from build123d import *

# Parameters (mm, degrees)
SKETCH1_W           = 186.97
SKETCH1_H           = 23
BOSS_EXTRUDE1_DEPTH = 4
SKETCH2_W           = 10
SKETCH2_H           = 23
BOSS_EXTRUDE2_DEPTH = 22
BOSS_EXTRUDE3_DEPTH = 8
CHAMFER1_SIZE       = 14.301043111
CHAMFER1_SIZE_2     = 12
CUT_EXTRUDE1_REACH  = 191.66
SKETCH4_W           = 9
SKETCH4_H           = 4.8
SKETCH4_H_2         = 4
SKETCH4_H_3         = 2.2
SKETCH4_W_2         = 3
SKETCH4_H_4         = 3
SKETCH5_W           = 6
SKETCH5_H           = 6
BOSS_EXTRUDE4_DEPTH = 9
CUT_EXTRUDE2_REACH  = 191.66
SKETCH6_W           = 6
SKETCH6_H           = 4
CUT_EXTRUDE3_REACH  = 192.165
SKETCH7_W           = 3
SKETCH7_H           = 3
SKETCH8_W           = 16
SKETCH8_H           = 23
BOSS_EXTRUDE5_DEPTH = 14
CHAMFER2_SIZE       = 14
CHAMFER2_SIZE_2     = 16.105157701
SKETCH9_W           = 9
SKETCH9_H           = 9
CUT_EXTRUDE4_DEPTH  = 2


with BuildPart() as part:
    # Sketch1 → Boss-Extrude1 (new body)
    with BuildSketch(Plane(origin=(0, 0, 0), x_dir=(1, 0, 0), z_dir=(0, 1, 0))):
        with Locations((93.485, 11.5)):
            Rectangle(SKETCH1_W, SKETCH1_H)
    extrude(amount=BOSS_EXTRUDE1_DEPTH)

    # Sketch2 → Boss-Extrude2 (add)
    with BuildSketch(Plane.XZ):
        with Locations((172.97, -11.5)):
            Rectangle(SKETCH2_W, SKETCH2_H)
    extrude(amount=BOSS_EXTRUDE2_DEPTH)

    # Sketch3 → Boss-Extrude3 (add)
    with BuildSketch(Plane.XZ):
        Polygon((167.97, 0), (38.01, 0), (38.01, -8), (38.01, -23), (62.01, -23), (62.01, -8), (167.97, -8), align=None)
    extrude(amount=BOSS_EXTRUDE3_DEPTH)

    # Chamfer1
    # the kernel refuses this chamfer: 14.301043111, 12 mm, written as the material it adds along each edge
    with BuildSketch(Plane(origin=(167.97, -8, -8), x_dir=(0.024939322090235156, -0.9996889667359941, 0), z_dir=(0, 0, 1))) as chamfer1_piece_1_section:
        Polygon((CHAMFER1_SIZE * 0.999688966745, -CHAMFER1_SIZE * 0.0249393220905), (-CHAMFER1_SIZE_2 * 0.0249393220902, -CHAMFER1_SIZE_2 * 0.999688966736), (0, 0), align=None)
    chamfer1_piece_1 = extrude(amount=8, mode=Mode.PRIVATE)
    chamfer1_piece_1 = split(chamfer1_piece_1, bisect_by=Plane(origin=(164.021429924, -22, -4), z_dir=(0, 1, 0)), keep=Keep.TOP, mode=Mode.PRIVATE)
    add(chamfer1_piece_1)

    # Sketch4 → Cut-Extrude1 (cut, up to next)
    with BuildSketch(Plane.XZ, mode=Mode.PRIVATE) as cut_extrude1_sk1:
        with Locations((182.47, -10.6)):
            Rectangle(SKETCH4_W, SKETCH4_H)
    cut_extrude1_tool1 = extrude(cut_extrude1_sk1.sketch, amount=-CUT_EXTRUDE1_REACH, mode=Mode.PRIVATE) & part.part
    # Sketch4 → Cut-Extrude1 (cut, up to next)
    with BuildSketch(Plane.XZ, mode=Mode.PRIVATE) as cut_extrude1_sk2:
        with Locations((182.47, -21)):
            Rectangle(SKETCH4_W, SKETCH4_H_2)
    cut_extrude1_tool2 = extrude(cut_extrude1_sk2.sketch, amount=-CUT_EXTRUDE1_REACH, mode=Mode.PRIVATE) & part.part
    # Sketch4 → Cut-Extrude1 (cut, up to next)
    with BuildSketch(Plane.XZ, mode=Mode.PRIVATE) as cut_extrude1_sk3:
        with Locations((182.47, -1.1)):
            Rectangle(SKETCH4_W, SKETCH4_H_3)
    cut_extrude1_tool3 = extrude(cut_extrude1_sk3.sketch, amount=-CUT_EXTRUDE1_REACH, mode=Mode.PRIVATE) & part.part
    # Sketch4 → Cut-Extrude1 (cut, up to next)
    with BuildSketch(Plane.XZ, mode=Mode.PRIVATE) as cut_extrude1_sk4:
        with Locations((182.47, -16)):
            Rectangle(SKETCH4_W_2, SKETCH4_H_4)
    cut_extrude1_tool4 = extrude(cut_extrude1_sk4.sketch, amount=-CUT_EXTRUDE1_REACH, mode=Mode.PRIVATE) & part.part
    # Sketch4 → Cut-Extrude1 (cut, up to next)
    with BuildSketch(Plane.XZ, mode=Mode.PRIVATE) as cut_extrude1_sk5:
        with Locations((182.47, -5.2)):
            Rectangle(SKETCH4_W_2, SKETCH4_H_4)
    cut_extrude1_tool5 = extrude(cut_extrude1_sk5.sketch, amount=-CUT_EXTRUDE1_REACH, mode=Mode.PRIVATE) & part.part
    # Sketch4 → Cut-Extrude1 (cut, up to next)
    with BuildSketch(Plane.XZ, mode=Mode.PRIVATE) as cut_extrude1_sk6:
        with Locations((4.5, -1.1)):
            Rectangle(SKETCH4_W, SKETCH4_H_3)
    cut_extrude1_tool6 = extrude(cut_extrude1_sk6.sketch, amount=-CUT_EXTRUDE1_REACH, mode=Mode.PRIVATE) & part.part
    # Sketch4 → Cut-Extrude1 (cut, up to next)
    with BuildSketch(Plane.XZ, mode=Mode.PRIVATE) as cut_extrude1_sk7:
        with Locations((4.5, -5.2)):
            Rectangle(SKETCH4_W_2, SKETCH4_H_4)
    cut_extrude1_tool7 = extrude(cut_extrude1_sk7.sketch, amount=-CUT_EXTRUDE1_REACH, mode=Mode.PRIVATE) & part.part
    # Sketch4 → Cut-Extrude1 (cut, up to next)
    with BuildSketch(Plane.XZ, mode=Mode.PRIVATE) as cut_extrude1_sk8:
        with Locations((4.5, -10.6)):
            Rectangle(SKETCH4_W, SKETCH4_H)
    cut_extrude1_tool8 = extrude(cut_extrude1_sk8.sketch, amount=-CUT_EXTRUDE1_REACH, mode=Mode.PRIVATE) & part.part
    # Sketch4 → Cut-Extrude1 (cut, up to next)
    with BuildSketch(Plane.XZ, mode=Mode.PRIVATE) as cut_extrude1_sk9:
        with Locations((4.5, -16)):
            Rectangle(SKETCH4_W_2, SKETCH4_H_4)
    cut_extrude1_tool9 = extrude(cut_extrude1_sk9.sketch, amount=-CUT_EXTRUDE1_REACH, mode=Mode.PRIVATE) & part.part
    # Sketch4 → Cut-Extrude1 (cut, up to next)
    with BuildSketch(Plane.XZ, mode=Mode.PRIVATE) as cut_extrude1_sk10:
        with Locations((4.5, -21)):
            Rectangle(SKETCH4_W, SKETCH4_H_2)
    cut_extrude1_tool10 = extrude(cut_extrude1_sk10.sketch, amount=-CUT_EXTRUDE1_REACH, mode=Mode.PRIVATE) & part.part
    add(cut_extrude1_tool1.solids().sort_by_distance((182.47, 0, -10.6))[0], mode=Mode.SUBTRACT)
    add(cut_extrude1_tool2.solids().sort_by_distance((182.47, 0, -21))[0], mode=Mode.SUBTRACT)
    add(cut_extrude1_tool3.solids().sort_by_distance((182.47, 0, -1.1))[0], mode=Mode.SUBTRACT)
    add(cut_extrude1_tool4.solids().sort_by_distance((182.47, 0, -16))[0], mode=Mode.SUBTRACT)
    add(cut_extrude1_tool5.solids().sort_by_distance((182.47, 0, -5.2))[0], mode=Mode.SUBTRACT)
    add(cut_extrude1_tool6.solids().sort_by_distance((4.5, 0, -1.1))[0], mode=Mode.SUBTRACT)
    add(cut_extrude1_tool7.solids().sort_by_distance((4.5, 0, -5.2))[0], mode=Mode.SUBTRACT)
    add(cut_extrude1_tool8.solids().sort_by_distance((4.5, 0, -10.6))[0], mode=Mode.SUBTRACT)
    add(cut_extrude1_tool9.solids().sort_by_distance((4.5, 0, -16))[0], mode=Mode.SUBTRACT)
    add(cut_extrude1_tool10.solids().sort_by_distance((4.5, 0, -21))[0], mode=Mode.SUBTRACT)

    # Sketch5 → Boss-Extrude4 (add)
    with BuildSketch(Plane(origin=(177.97, 0, 0), x_dir=(0, 0, -1), z_dir=(1, 0, 0))):
        with Locations((11.2, -9)):
            Rectangle(SKETCH5_W, SKETCH5_H)
    extrude(amount=BOSS_EXTRUDE4_DEPTH)

    # Sketch6 → Cut-Extrude2 (cut, up to next)
    with BuildSketch(Plane(origin=(0, 0, -23), x_dir=(-1, 0, 0), z_dir=(0, 0, -1)), mode=Mode.PRIVATE) as cut_extrude2_sk1:
        with Locations((-55.01, -2)):
            Rectangle(SKETCH6_W, SKETCH6_H)
    cut_extrude2_tool1 = extrude(cut_extrude2_sk1.sketch, amount=-CUT_EXTRUDE2_REACH, mode=Mode.PRIVATE) & part.part
    # Sketch6 → Cut-Extrude2 (cut, up to next)
    with BuildSketch(Plane(origin=(0, 0, -23), x_dir=(-1, 0, 0), z_dir=(0, 0, -1)), mode=Mode.PRIVATE) as cut_extrude2_sk2:
        with Locations((-45.01, -2)):
            Rectangle(SKETCH6_W, SKETCH6_H)
    cut_extrude2_tool2 = extrude(cut_extrude2_sk2.sketch, amount=-CUT_EXTRUDE2_REACH, mode=Mode.PRIVATE) & part.part
    add(cut_extrude2_tool1.solids().sort_by_distance((55.01, -2, -23))[0], mode=Mode.SUBTRACT)
    add(cut_extrude2_tool2.solids().sort_by_distance((45.01, -2, -23))[0], mode=Mode.SUBTRACT)

    # Sketch7 → Cut-Extrude3 (cut, up to next)
    with BuildSketch(Plane(origin=(0, 4, 0), x_dir=(1, 0, 0), z_dir=(0, 1, 0)), mode=Mode.PRIVATE) as cut_extrude3_sk1:
        with Locations((45.01, 11.5)):
            Rectangle(SKETCH7_W, SKETCH7_H)
    cut_extrude3_tool1 = extrude(cut_extrude3_sk1.sketch, amount=-CUT_EXTRUDE3_REACH, mode=Mode.PRIVATE) & part.part
    # Sketch7 → Cut-Extrude3 (cut, up to next)
    with BuildSketch(Plane(origin=(0, 4, 0), x_dir=(1, 0, 0), z_dir=(0, 1, 0)), mode=Mode.PRIVATE) as cut_extrude3_sk2:
        with Locations((55.01, 11.5)):
            Rectangle(SKETCH7_W, SKETCH7_H)
    cut_extrude3_tool2 = extrude(cut_extrude3_sk2.sketch, amount=-CUT_EXTRUDE3_REACH, mode=Mode.PRIVATE) & part.part
    add(cut_extrude3_tool1.solids().sort_by_distance((45.01, 4, -11.5))[0], mode=Mode.SUBTRACT)
    add(cut_extrude3_tool2.solids().sort_by_distance((55.01, 4, -11.5))[0], mode=Mode.SUBTRACT)

    # Sketch8 → Boss-Extrude5 (add)
    with BuildSketch(Plane.XZ):
        with Locations((17, -11.5)):
            Rectangle(SKETCH8_W, SKETCH8_H)
    extrude(amount=BOSS_EXTRUDE5_DEPTH)

    # Chamfer2
    # the kernel refuses this chamfer: 16.105157701, 14 mm, written as the material it takes off along each edge
    with BuildSketch(Plane(origin=(25, -14, 41.491821244), x_dir=(0.033690971337926715, 0.9994322980824198, 0), z_dir=(0, 0, -1))) as chamfer2_piece_1_section:
        Polygon((CHAMFER2_SIZE * 0.999432298082, -CHAMFER2_SIZE * 0.0336909713379), (-CHAMFER2_SIZE_2 * 0.0336909713381, -CHAMFER2_SIZE_2 * 0.999432298088), (0, 0), align=None)
    chamfer2_piece_1 = extrude(amount=105.983642488, mode=Mode.PRIVATE)
    chamfer2_piece_1 = split(chamfer2_piece_1, bisect_by=Plane(origin=(19.65817275, 0, -11.5), z_dir=(0, -1, 0)), keep=Keep.TOP, mode=Mode.PRIVATE)
    add(chamfer2_piece_1, mode=Mode.SUBTRACT)

    # Sketch9 → Cut-Extrude4 (cut)
    with BuildSketch(Plane(origin=(0, 4, 0), x_dir=(1, 0, 0), z_dir=(0, 1, 0))):
        with Locations((45.01, 11.5)):
            Rectangle(SKETCH9_W, SKETCH9_H)
        with Locations((55.01, 11.5)):
            Rectangle(SKETCH9_W, SKETCH9_H)
    extrude(amount=-CUT_EXTRUDE4_DEPTH, mode=Mode.SUBTRACT)


solid = part.part
Check sheet for the modelled part. Datum: model origin and axes. Units: mm. A direction names the side the tool comes from. Give positions to 0.01 mm unless a question says otherwise; leave off trailing zeros. Loops run counter-clockwise (first coordinate to the right, second up) from the corner with the lowest first, then second, coordinate; pieces in that order, holes last. Notation, with made-up numbers: M 58.5,87.5 L 92.5,87.5 A20 cw 92.5,102.5 Z; hole C -7.5,27.5 d4. An arc over 180 degrees is marked long. Use a Markdown table: item, result. Add a question column.
Q1. Tool access check on faces 5 (the flat face through (182, 2, -19)), 6 (the flat face through (83, -8, -6)), 7 (the flat face through (182, 2, -3.7)). Record the directions out of +Z, -Z, +X, -X, +Y, -Y that give a thin tool (end or side, any length) a straight path to the whole face; none if there is none.
Q2. Scan lines: line 1 along X through (y, z) = (-5.75, -10); line 2 along X through (y, z) = (1.5, -10.25); line 3 along X through (y, z) = (-1.25, -8.25). Record each from-to range of solid material in increasing order. Write a range as [from, to].
Q3. Sectioned sample at B-B, the plane x = 122. Record the cut outline in (y, z), then the cut area to 3 significant figures.
Q4. Go/stop test with flat-tipped pins: pin 1 (7.5 mm diameter, centred on x = 137, z = -15, fed in from -Y); pin 2 (1 mm diameter, centred on x = 20, y = -5.5, fed in from -Z); pin 3 (0.9 mm diameter, centred on x = 5, y = 3, fed in from +Z); pin 4 (1.5 mm diameter, centred on x = 182.5, y = 2, fed in from -Z). Record where each tip stops, or that it passes through.
Q5. Sectioned sample at C-C, the plane y = -20. Record the cut outline in (x, z).
Q6. Mould release check, pull along Y, two halves, no side actions. Record for faces 1 (the flat face through (31, 0, -12)), 2 (the flat face through (182, -6, -11)), 3 (the flat face through (48.01, -2, -12)), 4 (the flat face through (180.97, 2, -5)): pulls with the +Y half, pulls with the -Y half, needs draft (parallel to the pull), parting line crosses it, or undercut.
Q7. Sectioned sample at A-A, the plane z = -21. Record the cut outline in (x, y), then the cut area to 3 significant figures.
Q8. Sectioned sample at D-D, the plane x = 30. Record the cut outline in (y, z).
Verdict:
| question | item | result |
|---|---|---|
| 1 | face 5 | -Z, +X, +Y, -Y |
| 1 | face 6 | +Z, -Z, -Y |
| 1 | face 7 | +Y, -Y |
| 2 | line 1 | [9, 18.39], [38.01, 62.01], [167.97, 177.97] |
| 2 | line 2 | [9, 43.51], [46.51, 53.51], [56.51, 177.97] |
| 2 | line 3 | [9, 23.56], [38.01, 42.01], [48.01, 52.01], [58.01, 62.01], [167.97, 177.97] |
| 3 | outline | M -8,-8 L 0,-8 L 0,-23 L 4,-23 L 4,0 L -8,0 Z |
| 3 | area | 156 mm^2 |
| 4 | pin 1 | y = 0 |
| 4 | pin 2 | through |
| 4 | pin 3 | z = -2.2 |
| 4 | pin 4 | z = -19 |
| 5 | outline | M 166.04,-8 L 167.97,-8 L 167.97,-23 L 177.97,-23 L 177.97,0 L 166.04,0 Z |
| 6 | face 1 | pulls with the -Y half |
| 6 | face 2 | undercut |
| 6 | face 3 | undercut |
| 6 | face 4 | needs draft |
| 7 | outline | M 9,-13.91 L 25,0 L 38.01,0 L 38.01,-8 L 62.01,-8 L 62.01,0 L 167.97,0 L 167.97,-22 L 177.97,-22 L 177.97,4 L 9,4 Z; hole M 42.01,-4 L 48.01,-4 L 48.01,0 L 42.01,0 Z; hole M 52.01,-4 L 58.01,-4 L 58.01,0 L 52.01,0 Z |
| 7 | area | 1,150 mm^2 |
| 8 | outline | M 0,-23 L 4,-23 L 4,0 L 0,0 Z |
